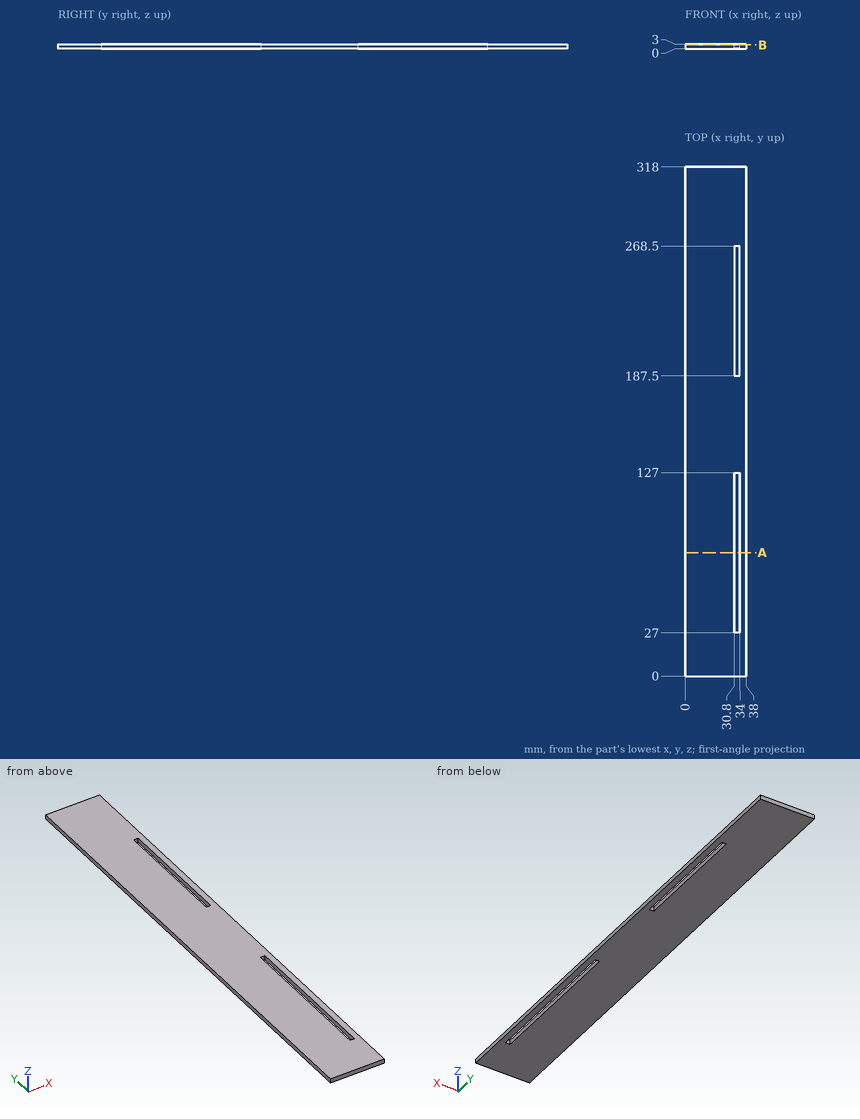
For this review, use the dimensioned drawing (mm, ordinates from the lowest corner) and the shaded views. Coordinates: 2 decimals unless noted, no trailing zeros. Loops run counter-clockwise (first coordinate to the right, second up) from the corner with the lowest first, then second, coordinate; pieces in that order, holes last. Notation, with made-up numbers: M 12,66.5 L 56,66.5 A23 ccw 56,83.5 Z; hole C -2,22.25 d8. An arc over 180 degrees is marked long. Answer as CSV lines item,"result".
Item 1: Add section A-A on y = 77. State the section outline as (x, z) points.
Answer list:
outline,"M 0,0 L 30.8,0 L 30.8,3 L 0,3 Z; M 34,0 L 38,0 L 38,3 L 34,3 Z"
Item 2: For P1, Ø10, axis at x = 24.5, y = 57.5, coming from the -Z side, flat-tipped, find the tip position at first contact; note if it passes through.
Answer list:
P1,"z = 0"
Item 3: For probe 1 along Y at (x, z) = (31, 0.4); probe 2 along X at (y, z) = (122, 0.85), list the stretches that pass through material, from the lowest coordinate up.
Answer list:
probe 1,"0 to 27, 127 to 187.5, 268.5 to 318"
probe 2,"0 to 30.8, 34 to 38"
Item 4: Add section B-B on z = 2.5. State the section outline as (x, y) points, plus the area to 3 significant figures.
Answer list:
outline,"M 0,0 L 38,0 L 38,318 L 0,318 Z; hole M 30.8,27 L 34,27 L 34,127 L 30.8,127 Z; hole M 30.8,187.5 L 34,187.5 L 34,268.5 L 30.8,268.5 Z"
area,"11,500 mm²"
